Part print with two shaded views. Sizes in mm from the minimum x, y, z corner. Give positions to 0.01 mm unless a question says otherwise; leave off trailing zeros. Loops run counter-clockwise (first coordinate to the right, second up) from the corner with the lowest first, then second, coordinate; pieces in that order, holes last. Notation, with made-up numbers: M 45.25,85.5 L 68.25,85.5 A29 cw 68.25,109.5 Z; hole C 4.25,21 d7. An arc over 180 degrees is marked long. Answer in a Markdown table with one row per item.
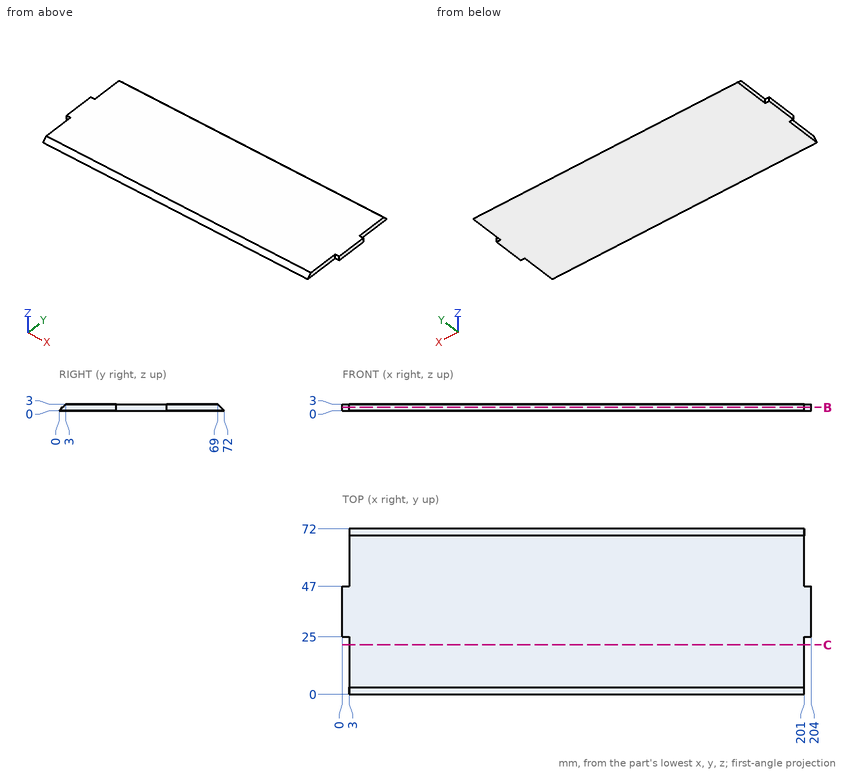
Q1. Saw through at B-B (z = 1.5). Give the cut face in (x, y).
Reported:
| item | result |
|---|---|
| outline | M 0,25 L 3,25 L 3,1.5 L 201,1.5 L 201,25 L 204,25 L 204,47 L 201,47 L 201,70.5 L 3,70.5 L 3,47 L 0,47 Z |
Q2. Drop flat-ended pins along their axis: pin 1 (0.9 mm diameter, centred on y = 11, z = 1, fed in from +X); pin 2 (1.5 mm diameter, centred on x = 102, z = 2, fed in from -Y); pin 3 (0.9 mm diameter, centred on x = 203, z = 1, fed in from +Y). Give the stop position or say it passes through.
Reported:
| item | result |
|---|---|
| pin 1 | x = 201 |
| pin 2 | y = 1.25 |
| pin 3 | y = 47 |
Q3. Saw through at C-C (y = 21.5). Give the cut face in (x, z), and give its area (3 significant figures).
Reported:
| item | result |
|---|---|
| outline | M 3,0 L 201,0 L 201,3 L 3,3 Z |
| area | 594 mm² |
Q4. Probe probe 1 along X at (y, z) = (55.5, 1.4); probe 2 along Y at (x, z) = (170, 2.05); probe 3 along Y at (x, z) = (122.5, 2.6). List the from-to ranges inside material, lowest first.
Reported:
| item | result |
|---|---|
| probe 1 | 3 to 201 |
| probe 2 | 2.05 to 69.95 |
| probe 3 | 2.6 to 69.4 |
